from build123d import *

# Parameters (mm, degrees)
CROQUIS1_R              = 1.5
SALIENTE_EXTRUIR1_DEPTH = 3


with BuildPart() as part:
    # Croquis1 → Saliente-Extruir1 (new body)
    with BuildSketch(Plane(origin=(0, 0, 0), x_dir=(0, 0, -1), z_dir=(1, 0, 0))):
        with BuildLine():
            ThreePointArc((-5, 0), (2.011533945, -4.57752457), (3.381492475, 3.683138423))
            ThreePointArc((3.381492475, 3.683138423), (-1.096196525, 75), (3.381492475, 146.316861577))
            ThreePointArc((3.381492475, 146.316861577), (2.011533945, 154.57752457), (-5, 150))
            ThreePointArc((-5, 150), (-9.607489913, 75), (-5, 0))
        make_face()
        with Locations((0, 150)):
            Circle(CROQUIS1_R, mode=Mode.SUBTRACT)
        Circle(CROQUIS1_R, mode=Mode.SUBTRACT)
    extrude(amount=SALIENTE_EXTRUIR1_DEPTH)


solid = part.part
Can you work these out from the model? Positions are in its coordinate system, mm. Coordinates: 2 decimals unless noted, no trailing zeros. Write each loop counter-clockwise with the first axis right and the second up, starting at its lowest first coordinate (ties: lowest second). Pieces come first, ordered by that corner, then holes. Notation, with made-up numbers: (-13.75, -25) - (3.25, -25) arc R19 ccw to (3.25, -2) - close; hole circle Ø4 at (-12.5, 87.25). An arc over 180 degrees is marked (long way). Return JSON: item names as keys, results as strings. Group by question number.
Item 1: If we section it at A-A (x = 1.8): Write out the boundary of the cut face in (y, z).
Item 2: We'd pull the mould along Y, two halves only. Please class faces 1 (the face through (3, 76, 4)), 2 (the face through (1.479, 76.053, 9.607)), 3 (the face through (1.479, 151.487, 0.195)), 4 (the face through (1.48, 0.07, 1.5)): pulls with the +Y half, pulls with the -Y half, needs draft (parallel to the pull), parting line crosses it, or undercut.
Item 3: If we section it at B-B (y = 23.5): Write out the boundary of the cut face in (x, z).
Item 4: I'm going to push a flat-ended pin straight in: pin 1 Ø2.5 at (y, z) = (0, 0) entering from -X. Where does the tip first touch, or does it pass through?
Item 5: Please list where these lines run through material, in increasing order: probe 1 along Z at (x, y) = (1.45, 150); probe 2 along Y at (x, z) = (0.65, -3.5); probe 3 along Z at (x, y) = (0.7, 140).
Return value:
{
 "1": {"outline": "(0, 5) arc R5 ccw (long way) to (3.68, -3.38) arc R570.18 cw to (146.32, -3.38) arc R5 ccw (long way) to (150, 5) arc R612.72 ccw to start; hole circle Ø3 at (0, 0); hole circle Ø3 at (150, 0)"},
 "2": {"face 1": "needs draft", "face 2": "parting line crosses it", "face 3": "undercut", "face 4": "undercut"},
 "3": {"outline": "(0, -1.23) - (3, -1.23) - (3, 7.44) - (0, 7.44) - close"},
 "4": {"pin 1": "passes through"},
 "5": {"probe 1": "z = -5 to -1.5, 1.5 to 5", "probe 2": "y = -3.57 to 3.57, 146.43 to 153.57", "probe 3": "z = -2.62 to 6.15"}
}
